Geometry check sheet. Reference: the model listing, model coordinates, mm. Face numbers are marked on the shaded views. A direction names the side the tool comes from. Give positions to 0.01 mm unless a question says otherwise; leave off trailing zeros. Write each loop counter-clockwise with the first axis right and the second up, starting at its lowest first coordinate (ties: lowest second). Pieces come first, ordered by that corner, then holes. Notation, with made-up numbers: (72, -16) -> (116, -16) arc R29 ccw to (116, 23) -> close; hole circle Ø8 at (20, -35). An arc over 180 degrees is marked (long way). One line per item, written item: value.
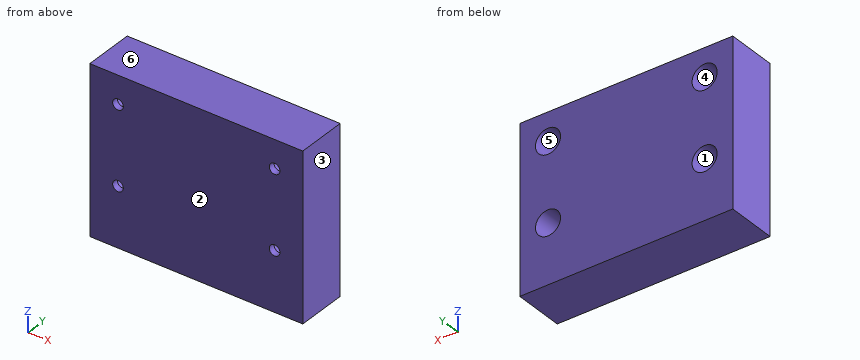
Autodesk Inventor part; units mm, degrees
ref_plane "YZ Plane" through (0, 0, 0) normal (1, 0, 0) x (0, 1, 0)
ref_plane "XZ Plane" through (0, 0, 0) normal (0, 1, 0) x (-1, 0, 0)
ref_plane "XY Plane" through (0, 0, 0) normal (0, 0, 1) x (1, 0, 0)
sketch "Sketch1" plane through (0, 0, 0) normal (0, 1, 0) x (-1, 0, 0)
  line L0 (7.4046, 11.4154) -> (-60.5954, 11.4154)
  line L1 (-60.5954, 11.4154) -> (-60.5954, -41.5846)
  line L2 (-60.5954, -41.5846) -> (7.4046, -41.5846)
  line L3 (7.4046, -41.5846) -> (7.4046, 11.4154)
  point P0 (0, 0)
  dimension "d0" = 68
  dimension "d1" = 53
extrude "Extrusion1" add sketch "Sketch1" along normal blind 16
sketch "Sketch2" plane through (0, 16, 0) normal (0, 1, 0) x (1, 0, 0)
  circle A0 centre (1.5954, -2.4154) radius 4
  circle A1 centre (1.5954, 22.5846) radius 4
  circle A2 centre (51.5954, 22.5846) radius 4
  circle A3 centre (51.5954, -2.4154) radius 4
  line L0 (-7.4046, 41.5846) -> (-7.4046, -11.4154)
  line L1 (-7.4046, -11.4154) -> (60.5954, -11.4154)
  point P0 (0, 0)
  dimension "d4" = 8
  dimension "d5" = 8
  dimension "d6" = 8
  dimension "d7" = 8
  dimension "d8" = 50
  dimension "d9" = 25
  dimension "d10" = 9
  dimension "d11" = 9
extrude "Extrusion2" cut sketch "Sketch2" against normal blind 14
sketch "Sketch3" plane through (1.5954, 2, 2.4154) normal (0, 1, 0) x (1, 0, 0)
  circle A0 centre (0, 0) radius 4
  circle A1 centre (0, 0) radius 1.7
  circle A2 centre (0, 25) radius 4
  circle A3 centre (0, 25) radius 1.7
  circle A4 centre (50, 25) radius 4
  circle A5 centre (50, 25) radius 1.7
  circle A6 centre (50, 0) radius 4
  circle A7 centre (50, 0) radius 1.7
  point P0 (-1.5954, 2.4154)
  dimension "d14" = 3.4
  dimension "d15" = 3.4
  dimension "d16" = 3.4
  dimension "d17" = 3.4
extrude "Extrusion3" cut sketch "Sketch3" against normal through all contours A1 | A3 | A5 | A7
properties part number "bottomMotorMount"
1) Scan lines: probe 1 along Z at (x, y) = (54, 6); probe 2 along X at (y, z) = (14.75, -24.5); probe 3 along Y at (x, z) = (2, 6). Record each from-to range of solid material in increasing order.
Verdict:
probe 1: -41.58 to -25.78, -19.39 to -0.78, 5.61 to 11.42
probe 2: -7.4 to -1.92, 5.11 to 48.08, 55.11 to 60.6
probe 3: 0 to 2
2) Sectioned sample at B-B on y = 13.75. Record the cut outline in (x, z).
Verdict:
outline: (-7.4, -41.58) -> (60.6, -41.58) -> (60.6, 11.42) -> (-7.4, 11.42) -> close; hole circle Ø8 at (1.6, -22.58); hole circle Ø8 at (1.6, 2.42); hole circle Ø8 at (51.6, -22.58); hole circle Ø8 at (51.6, 2.42)
3) Mould release check, pull along X, two halves, no side actions. Record for the marked faces 1, 2, 3 and 4: released by +X, released by -X, zero draft, split by the parting line, or undercut.
Verdict:
face 1: undercut
face 2: zero draft
face 3: released by +X
face 4: undercut
4) Sectioned sample at A-A on x = 1.5. Record the cut outline in (y, z).
Verdict:
outline: (0, -41.58) -> (16, -41.58) -> (16, -26.58) -> (2, -26.58) -> (2, -24.28) -> (0, -24.28) -> close; (0, -20.89) -> (2, -20.89) -> (2, -18.59) -> (16, -18.59) -> (16, -1.58) -> (2, -1.58) -> (2, 0.72) -> (0, 0.72) -> close; (0, 4.11) -> (2, 4.11) -> (2, 6.41) -> (16, 6.41) -> (16, 11.42) -> (0, 11.42) -> close
5) Depth check by flat-ended pin: pin 1 Ø4 at (x, z) = (1.5, -23.5) entering from +Y; pin 2 Ø2.5 at (x, z) = (1.6, 2.42) entering from -Y. Enter the tip coordinate at first touch or a pass-through.
Verdict:
pin 1: y = 2
pin 2: through
6) Tool access check on the marked faces 5 and 6. Record the directions out of +Z, -Z, +X, -X, +Y, -Y that give a thin tool (end or side, any length) a straight path to the whole face; none if there is none.
Verdict:
face 5: +Y
face 6: +Z, +X, -X, +Y, -Y
